Print and shaded views of the part. All mm, measured from the part's lowest x, y and z. A direction names the side the tool comes from. Round coordinates to 2 decimals unless told otherwise and drop trailing zeros. Order: outer loops, then holes, each group sorted by start corner. A loop starts at its lowest first (then second) coordinate and runs counter-clockwise, first axis right, second up. Notation, with made-up numbers: (60, 65.5) -> (118, 65.5) arc R16 ccw to (118, 83.5) -> close; hole circle Ø6 at (34, -18). An arc over 180 degrees is marked (long way). Answer as CSV lines item,"result". Start each with the question number.
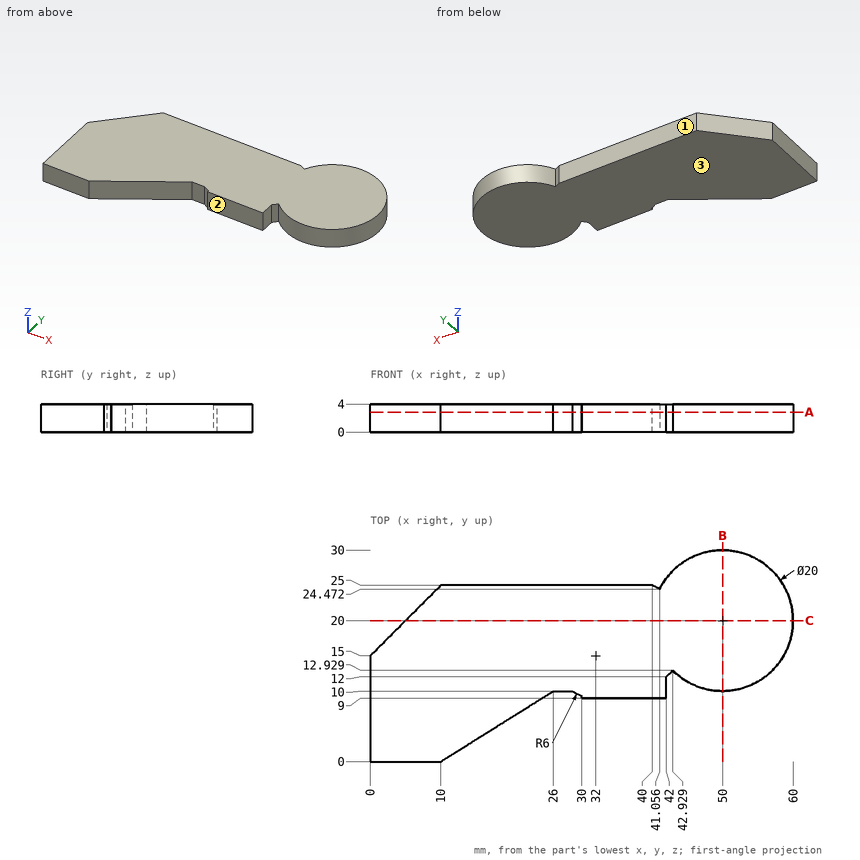
Item 1: Tool access for the marked faces 1, 2 and 3: list every direction of +Z, -Z, +X, -X, +Y, -Y with a clear straight run to the whole face (end or side of a thin tool).
Item 2: Band-saw the part on C-C, the plane y = 20. Give the cut face in (x, z).
Item 3: Pin check, flat tips, straight feed: pin 1 (2 mm diameter, centred on x = 16.5, z = 0.5, fed in from -Y); pin 2 (1 mm diameter, centred on y = 26.5, z = 2.5, fed in from -X); pin 3 (1.5 mm diameter, centred on x = 13, z = 2.5, fed in from -Y). Stop position of each tip, or through.
Item 4: Band-saw the part on B-B, the plane x = 50. Give the cut face in (y, z), and give its area (3 significant figures).
Item 5: Probe line 1 (Y direction, x = 35, z = 3.3); line 2 (X direction, y = 20.5, z = 3); line 3 (X direction, y = 6.25, z = 2.35). List the from-to ranges inside material, lowest first.
Item 6: Band-saw the part on A-A, the plane z = 2.85. Give the cut face in (x, y), and give its area (3 significant figures).
Values:
1,face 1,"+Z, -Z, -X, +Y"
1,face 2,"+Z, -Z, +X, -Y"
1,face 3,"-Z, +X, -X, +Y, -Y"
2,outline,"(5, 0) -> (60, 0) -> (60, 4) -> (5, 4) -> close"
3,pin 1,"y = 3.44"
3,pin 2,"x = 42"
3,pin 3,"y = 1.41"
4,outline,"(10, 0) -> (30, 0) -> (30, 4) -> (10, 4) -> close"
4,area,"80.0 mm²"
5,line 1,"9 to 25"
5,line 2,"5.5 to 59.99"
5,line 3,"0 to 20"
6,outline,"(0, 0) -> (10, 0) -> (26, 10) -> (28.68, 10) arc R6 ccw to (30, 9.34) -> (30, 9) -> (42, 9) -> (42, 12) -> (42.93, 12.93) arc R10 ccw (long way) to (41.06, 24.47) -> (40, 25) -> (10, 25) -> (0, 15) -> close"
6,area,"1,070 mm²"
